Check sheet for the modelled part. Datum: model origin and axes. Units: mm. A direction names the side the tool comes from. Round coordinates to 2 decimals unless told otherwise and drop trailing zeros. Write each loop counter-clockwise with the first axis right and the second up, starting at its lowest first coordinate (ties: lowest second). Pieces come first, ordered by that corner, then holes. Notation, with made-up numbers: M 26,77 L 36,77 A31 ccw 36,102 Z; hole C -35,50.5 d8. An arc over 180 degrees is marked long. Put each result on its own line as item: value.
```python
from build123d import *

# Parameters (mm, degrees)
F0_R     = 2
F1_DEPTH = 4
F3_DEPTH = 0.4
F4_SIZE  = 1


with BuildPart() as f1:
    # F0 (on Top) → F1 (new body)
    with BuildSketch(Plane.XY):
        Polygon((12, 12), (120, 12), (120, 27), (27, 27), (27, 60), (12, 60), align=None)
        Polygon((0, 60), (0, 0), (120, 0), (120, 12), (12, 12), (12, 60), align=None)
        with Locations((25, 6)):
            Circle(F0_R, mode=Mode.SUBTRACT)
        with Locations((95, 6)):
            Circle(F0_R, mode=Mode.SUBTRACT)
        with Locations((6, 50)):
            Circle(F0_R, mode=Mode.SUBTRACT)
    extrude(amount=F1_DEPTH)

    # F2 (on face) → F3 (join)
    with BuildSketch(Plane.XY.offset(4)):
        Polygon((27, 60), (12, 60), (12, 12), (120, 12), (120, 27), (27, 27), align=None)
    extrude(amount=F3_DEPTH)

    # F4
    f4_edges = [f1.edges().sort_by_distance(p)[0] for p in [
        (120, 13.5, 0),
        (13.5, 60, 0),
        (60, 0, 0),
        (0, 30, 0),
    ]]
    chamfer(f4_edges, length=F4_SIZE)


solid = f1.part
```
1. Cross-section at D-D (x = 95). Enter the section's corners in (y, z), then the cut area to 3 significant figures.
Computed values:
outline: M 0,1 L 1,0 L 4,0 L 4,4 L 0,4 Z; M 8,0 L 27,0 L 27,4.4 L 12,4.4 L 12,4 L 8,4 Z
area: 97.5 mm2
2. Depth check by flat-ended pin: pin 1 Ø1 at (x, z) = (31, 3.5) entering from +Y; pin 2 Ø2 at (y, z) = (44, 1.5) entering from +X; pin 3 Ø5 at (x, y) = (25, 6) entering from +Z. Enter the tip coordinate at first touch or a pass-through.
Computed values:
pin 1: stops at y = 27
pin 2: stops at x = 27
pin 3: stops at z = 4
3. Scan lines: probe 1 along Y at (x, z) = (25, 2); probe 2 along Y at (x, z) = (102.5, 2). Record each from-to range of solid material in increasing order.
Computed values:
probe 1: y = 0 to 4, 8 to 60
probe 2: y = 0 to 27
4. Release check for a two-part mould opening along Y. For faces 1 (the flat face through (46, 18, 0)), 2 (the flat face through (59, 0, 2)), 3 (the flat face through (14, 60, 3)), 4 (the cylindrical face through (96.908, 6.601, 1.972)) record: +Y half, -Y half, draft (parallel to the pull), parting line (faces both ways), or undercut.
Computed values:
face 1: draft
face 2: -Y half
face 3: +Y half
face 4: undercut
5. Cross-section at B-B (z = 2.5). Enter the section's corners in (x, y).
Computed values:
outline: M 0,0 L 120,0 L 120,27 L 27,27 L 27,60 L 0,60 Z; hole C 6,50 d4; hole C 25,6 d4; hole C 95,6 d4
6. Cross-section at A-A (x = 25). Enter the section's corners in (y, z).
Computed values:
outline: M 0,1 L 1,0 L 4,0 L 4,4 L 0,4 Z; M 8,0 L 59,0 L 60,1 L 60,4.4 L 12,4.4 L 12,4 L 8,4 Z
7. Cross-section at C-C (y = 32). Enter the section's corners in (x, z).
Computed values:
outline: M 0,1 L 1,0 L 27,0 L 27,4.4 L 12,4.4 L 12,4 L 0,4 Z
8. Access from +Z, -Z, +X, -X, +Y, -Y to the whole of each face (thin tool, end or side, straight path). Record for faces 5 (the flat face through (74, 27, 2)), 6 (the flat face through (120, 13, 3)).
Computed values:
face 5: +Z, -Z, +X, +Y
face 6: +Z, -Z, +X, +Y, -Y
